```python
from build123d import *

# Parameters (mm, degrees)
F0_R     = 3.175
F0_R_2   = 6.2865
F0_R_3   = 5.0419
F0_R_4   = 11.176
F1_DEPTH = 31.75


with BuildPart() as f1:
    # F0 (on Top) → F1 (new body)
    with BuildSketch(Plane.XY):
        with BuildLine():
            Line((-5.159375, 19.982173), (-40.878125, 10.759632))
            ThreePointArc((-40.878125, 10.759632), (-49.2125, 0), (-40.878125, -10.759632))
            Line((-40.878125, -10.759632), (-5.159375, -19.982173))
            ThreePointArc((-5.159375, -19.982173), (0, -20.6375), (5.159375, -19.982173))
            Line((5.159375, -19.982173), (40.878125, -10.759632))
            ThreePointArc((40.878125, -10.759632), (49.2125, 0), (40.878125, 10.759632))
            Line((40.878125, 10.759632), (5.159375, 19.982173))
            ThreePointArc((5.159375, 19.982173), (0, 20.6375), (-5.159375, 19.982173))
        make_face()
        with Locations((-12.7, -12.7)):
            Circle(F0_R, mode=Mode.SUBTRACT)
        with Locations((12.7, -12.7)):
            Circle(F0_R, mode=Mode.SUBTRACT)
        with Locations((-38.1, 0)):
            Circle(F0_R_2, mode=Mode.SUBTRACT)
        with Locations((-19.05, 0)):
            Circle(F0_R_3, mode=Mode.SUBTRACT)
        with Locations((-12.7, 12.7)):
            Circle(F0_R, mode=Mode.SUBTRACT)
        Circle(F0_R_4, mode=Mode.SUBTRACT)
        with Locations((19.05, 0)):
            Circle(F0_R_3, mode=Mode.SUBTRACT)
        with Locations((38.1, 0)):
            Circle(F0_R_2, mode=Mode.SUBTRACT)
        with Locations((12.7, 12.7)):
            Circle(F0_R, mode=Mode.SUBTRACT)
    extrude(amount=F1_DEPTH)


solid = f1.part
```
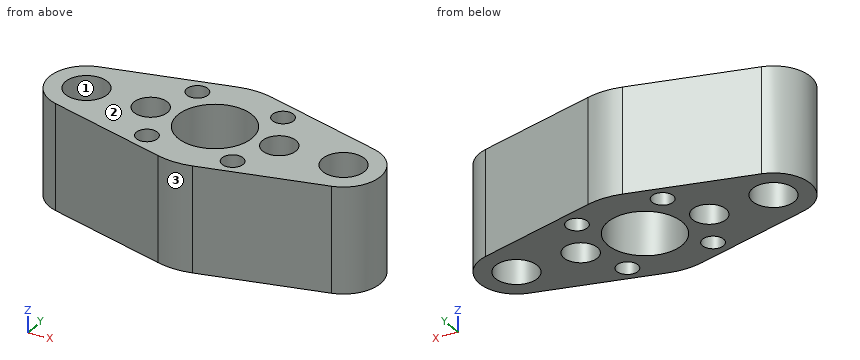
Work out the finished part from the listing and answer in its coordinate system (mm). Face numbers are marked on the shaded views. Coordinates: 2 decimals unless noted, no trailing zeros. Write each loop counter-clockwise with the first axis right and the second up, starting at its lowest first coordinate (ties: lowest second). Pieces come first, ordered by that corner, then holes.
Q1. Determine the mould class of the marked faces 1, 2 and 3 for opening direction Y: released by +Y, released by -Y, zero draft, split by the parting line, or undercut.
Q2. A cutting plane is placed at B-B, the plane z = 29. State how many separate pieces and enclosed holes the cut face has, then the cut area to 3 significant figures.
Q3. Each of these flat-tipped pins is pushed along its axis until it touches: pin 1 Ø1.5 at (x, y) = (-18.5, 12.5) entering from -Z; pin 2 Ø12 at (y, z) = (-11, 11.5) entering from +X; pin 3 Ø2 at (x, z) = (2, 9) entering from -Y; pin 4 Ø5 at (y, z) = (8.5, 15.5) entering from -X. Where does it stop, or does it pass through?
Q4. A cutting plane is placed at C-C, the plane x = 0. Give the vertices of the cut face in (y, z), then the cut area to 3 significant figures.
Q5. A cutting plane is placed at D-D, the plane x = 12.7. Give the vertices of the cut face in (y, z) (3 decimals).
Q6. A cutting plane is placed at A-A, the plane y = 0. Give the vertices of the cut face in (x, z), then the cut area to 3 significant figures.
Q7. Find the intervals of material crossed by line 1 (Y direction, x = 0, z = 19); line 2 (X direction, y = -0.5, z = 27.5); line 3 (X direction, y = -3.5, z = 3), in increasing order.
Findings below:
1. face 1: undercut
1. face 2: zero draft
1. face 3: released by -Y
2. separate pieces: 1
2. enclosed holes: 9
2. area: 1,960 mm2
3. pin 1: stops at z = 0
3. pin 2: stops at x = 48.02
3. pin 3: stops at y = -20.61
3. pin 4: stops at x = -47.45
4. outline: (-20.64, 0) - (-11.18, 0) - (-11.18, 31.75) - (-20.64, 31.75) - close; (11.18, 0) - (20.64, 0) - (20.64, 31.75) - (11.18, 31.75) - close
4. area: 601 mm2
5. outline: (-18.035, 0) - (-15.875, 0) - (-15.875, 31.75) - (-18.035, 31.75) - close; (-9.525, 0) - (9.525, 0) - (9.525, 31.75) - (-9.525, 31.75) - close; (15.875, 0) - (18.035, 0) - (18.035, 31.75) - (15.875, 31.75) - close
6. outline: (-49.21, 0) - (-44.39, 0) - (-44.39, 31.75) - (-49.21, 31.75) - close; (-31.81, 0) - (-24.09, 0) - (-24.09, 31.75) - (-31.81, 31.75) - close; (-14.01, 0) - (-11.18, 0) - (-11.18, 31.75) - (-14.01, 31.75) - close; (11.18, 0) - (14.01, 0) - (14.01, 31.75) - (11.18, 31.75) - close; (24.09, 0) - (31.81, 0) - (31.81, 31.75) - (24.09, 31.75) - close; (44.39, 0) - (49.21, 0) - (49.21, 31.75) - (44.39, 31.75) - close
6. area: 977 mm2
7. line 1: y = -20.64 to -11.18, 11.18 to 20.64
7. line 2: x = -49.2 to -44.37, -31.83 to -24.07, -14.03 to -11.16, 11.16 to 14.03, 24.07 to 31.83, 44.37 to 49.2
7. line 3: x = -48.65 to -43.32, -32.88 to -22.68, -15.42 to -10.61, 10.61 to 15.42, 22.68 to 32.88, 43.32 to 48.65
